Geometry check sheet. Reference: the model listing, model coordinates, mm. Face numbers are marked on the shaded views. Give positions to 0.01 mm unless a question says otherwise; leave off trailing zeros. Write each loop counter-clockwise with the first axis right and the second up, starting at its lowest first coordinate (ties: lowest second). Pieces come first, ordered by that corner, then holes. Notation, with made-up numbers: (-18, 12.25) - (-7, 12.25) arc R17 cw to (-7, 16.25) - close; hole circle Ø11 at (-26, 77). An arc over 180 degrees is marked (long way). Use a Markdown table: item, result.
```python
from build123d import *

# Parameters (mm, degrees)
BOSS_EXTRUDE1_DEPTH = 14
SKETCH3_R           = 4.125
CUT_EXTRUDE1_DEPTH  = 6
SKETCH5_R           = 1.125
CUT_EXTRUDE2_DEPTH  = 15
CUT_EXTRUDE5_DEPTH  = 6
CUT_EXTRUDE6_REACH  = 108.478
SKETCH16_R          = 1.6
BOSS_EXTRUDE2_START = 20
BOSS_EXTRUDE2_DEPTH = 20
BOSS_EXTRUDE3_DEPTH = 2.5
BOSS_EXTRUDE4_START = -34
BOSS_EXTRUDE4_DEPTH = 2.5


with BuildPart() as part:
    # Sketch1 → Boss-Extrude1 (new body)
    with BuildSketch(Plane(origin=(0, 0, 0), x_dir=(1, 0, 0), z_dir=(0, 1, 0))):
        with BuildLine():
            Line((47.5, -78.442713945), (47.5, -38.442713945))
            ThreePointArc((47.5, -38.442713945), (23.533579371, -5.900241558), (37.627970881, 31.977851779))
            Line((37.627970881, 31.977851779), (49.091933627, 57.755216031))
            Line((49.091933627, 57.755216031), (0, 0))
            Line((0, 0), (35.1, -73.422380253))
            Line((35.1, -73.422380253), (35.1, -93.442713945))
            Line((35.1, -93.442713945), (37.5, -93.442713945))
            Line((37.5, -93.442713945), (47.5, -93.442713945))
            Line((47.5, -93.442713945), (47.5, -78.442713945))
        make_face()
    extrude(amount=BOSS_EXTRUDE1_DEPTH)

    # Sketch3 → Cut-Extrude1 (cut)
    with BuildSketch(Plane.XZ):
        with BuildLine():
            Line((33.254958794, 84.403112572), (36.18509612, 92.428977457))
            Line((36.18509612, 92.428977457), (44.88509612, 92.428977457))
            Line((44.88509612, 92.428977457), (46.13509612, 88.028977457))
            Line((46.13509612, 88.028977457), (46.13509612, 70.028977457))
            Line((46.13509612, 70.028977457), (44.820911197, 53.062159312))
            ThreePointArc((44.820911197, 53.062159312), (40.059955227, 48.679043991), (35.34566343, 53.112310791))
            Line((35.34566343, 53.112310791), (33.254958794, 84.403112572))
        make_face()
        with Locations(Location((40.08509612, 83.428977457, 0), (0, 0, 90))):
            Circle(SKETCH3_R, mode=Mode.SUBTRACT)
    extrude(amount=-CUT_EXTRUDE1_DEPTH, mode=Mode.SUBTRACT)

    # Sketch5 → Cut-Extrude2 (cut)
    with BuildSketch(Plane.XZ.offset(-6)):
        with Locations(Location((40.08509612, 63.428977457, 0), (0, 0, 270))):
            Circle(SKETCH5_R)
        with Locations(Location((40.08509612, 58.928977457, 0), (0, 0, 270))):
            Circle(SKETCH5_R)
        with Locations(Location((40.08509612, 53.428977457, 0), (0, 0, 270))):
            Circle(SKETCH5_R)
    extrude(amount=-CUT_EXTRUDE2_DEPTH, mode=Mode.SUBTRACT)

    # Sketch15 → Cut-Extrude5 (cut)
    with BuildSketch(Plane(origin=(0, 6, 0), x_dir=(-1, 0, 0), z_dir=(0, -1, 0))):
        Polygon((-32.170978305, -71.382705183), (-57.86059863, -71.382705183), (-57.86059863, -110.098742661), (-30.980040887, -110.098742661), align=None)
    extrude(amount=CUT_EXTRUDE5_DEPTH, mode=Mode.SUBTRACT)

    # Sketch16 → Cut-Extrude6 (cut, up to next)
    with BuildSketch(Plane(origin=(0, 14, 0), x_dir=(1, 0, 0), z_dir=(0, 1, 0)), mode=Mode.PRIVATE) as cut_extrude6_sk1:
        with Locations(Location((40.08509612, -83.428977457, 0), (0, 0, 270))):
            Circle(SKETCH16_R)
    cut_extrude6_tool1 = extrude(cut_extrude6_sk1.sketch, amount=-CUT_EXTRUDE6_REACH, mode=Mode.PRIVATE) & part.part
    add(cut_extrude6_tool1.solids().sort_by_distance((40.085096, 14, 83.428977))[0], mode=Mode.SUBTRACT)

    # Sketch17 → Boss-Extrude2 (add)
    with BuildSketch(Plane(origin=(0, 0, 0), x_dir=(-1, 0, 0), z_dir=(0, -1, 0)).offset(BOSS_EXTRUDE2_START)):
        with BuildLine():
            Line((-37.627970881, 31.977851779), (-49.091933627, 57.755216031))
            Line((-49.091933627, 57.755216031), (0, 0))
            Line((0, 0), (-23.158323847, -48.442713945))
            Line((-23.158323847, -48.442713945), (-47.5, -48.442713945))
            Line((-47.5, -48.442713945), (-47.5, -38.442713945))
            ThreePointArc((-47.5, -38.442713945), (-23.533579371, -5.900241558), (-37.627970881, 31.977851779))
        make_face()
    extrude(amount=-BOSS_EXTRUDE2_DEPTH)

    # Sketch18 → Boss-Extrude3 (add)
    with BuildSketch(Plane(origin=(0, 14, 0), x_dir=(1, 0, 0), z_dir=(0, 1, 0))):
        Polygon((23.122023742, 27.202380873), (49.091933627, 57.755216031), (59.091933627, 57.755216031), (59.091933627, -38.442713945), (23.122023742, -38.442713945), align=None)
    extrude(amount=-BOSS_EXTRUDE3_DEPTH)

    # Sketch18<2> → Boss-Extrude4 (add)
    with BuildSketch(Plane(origin=(0, 14, 0), x_dir=(1, 0, 0), z_dir=(0, 1, 0)).offset(BOSS_EXTRUDE4_START)):
        Polygon((23.122023742, 27.202380873), (49.091933627, 57.755216031), (59.091933627, 57.755216031), (59.091933627, -38.442713945), (23.122023742, -38.442713945), align=None)
    extrude(amount=BOSS_EXTRUDE4_DEPTH)


solid = part.part
```
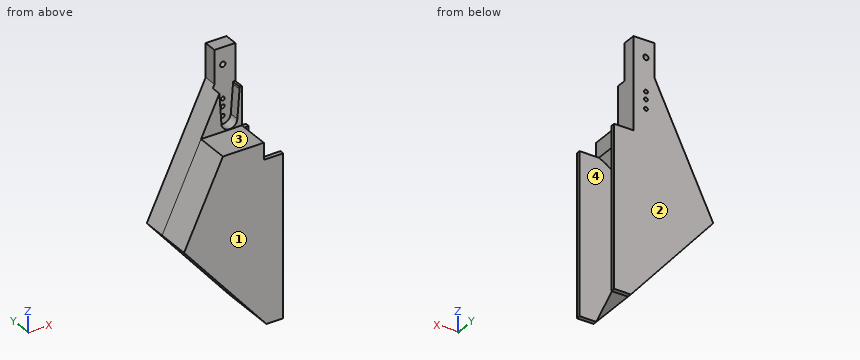
1) Depth check by flat-ended pin: P1, Ø1.8, axis at x = 40.09, z = 53.43, coming from the -Y side; P2, Ø6, axis at x = 9, y = 0.5, coming from the -Z side; P3, Ø1.1, axis at y = 2.5, z = 71, coming from the -X side; P4, Ø3.5, axis at x = 40.09, z = 63.43, coming from the -Y side. Enter the tip coordinate at first touch or a pass-through.
Working result:
| item | result |
|---|---|
| P1 | passes through |
| P2 | stops at z = -14.12 |
| P3 | stops at x = 33.68 |
| P4 | stops at y = 6 |
2) Material ranges on L1, parallel to Y at x = 43, z = 8; L2, parallel to Y at x = 45, z = 83; L3, parallel to Z at x = 32, y = -4, recorded low to high. Write a range as from..to.
Working result:
| item | result |
|---|---|
| L1 | y = -20..-17.5, 11.5..14 |
| L2 | y = 6..14 |
| L3 | z = -37.65..-26, 26..48.44 |
3) Section check A-A on x = 29. Record the boundary of the cut face in (y, z), then the cut area to 3 significant figures.
Working result:
| item | result |
|---|---|
| outline | (-20, -34.12) - (14, -34.12) - (14, 60.66) - (0, 60.66) - (0, 48.44) - (-20, 48.44) - close; hole (-17.5, -21.57) - (11.5, -21.57) - (11.5, 21.57) - (-17.5, 21.57) - close |
| area | 1,730 mm² |
4) Mould release check, pull along Y, two halves, no side actions. Record for the marked faces 1, 2, 3 and 4: pulls with the +Y half, pulls with the -Y half, needs draft (parallel to the pull), parting line crosses it, or undercut.
Working result:
| item | result |
|---|---|
| face 1 | pulls with the -Y half |
| face 2 | pulls with the +Y half |
| face 3 | needs draft |
| face 4 | undercut |
5) Section check D-D on x = 18. Record the boundary of the cut face in (y, z), then the cut area to 3 significant figures.
Working result:
| item | result |
|---|---|
| outline | (-20, -21.18) - (14, -21.18) - (14, 37.65) - (-20, 37.65) - close |
| area | 2,000 mm² |
6) Section check C-C on z = 6. Record the boundary of the cut face in (x, y).
Working result:
| item | result |
|---|---|
| outline | (2.87, -20) - (59.09, -20) - (59.09, -17.5) - (23.55, -17.5) - (23.55, 11.5) - (59.09, 11.5) - (59.09, 14) - (2.87, 14) - close |
7) Section check B-B on y = -9.5. Record the boundary of the cut face in (x, z), then the cut area to 3 significant figures.
Working result:
| item | result |
|---|---|
| outline | (0, 0) - (49.09, -57.76) - (37.63, -31.98) arc R42.5 cw to (47.5, 38.44) - (47.5, 48.44) - (23.16, 48.44) - close |
| area | 1,650 mm² |
